Geometry check sheet. Reference: the model listing, model coordinates, mm. A direction names the side the tool comes from. Coordinates: 2 decimals unless noted, no trailing zeros. Loops run counter-clockwise (first coordinate to the right, second up) from the corner with the lowest first, then second, coordinate; pieces in that order, holes last. Notation, with made-up numbers: (-3.75, -16.5) - (49.25, -16.5) arc R20 cw to (49.25, 21.5) - close; hole circle Ø2 at (46.25, -2.75). An arc over 180 degrees is marked (long way). Write each question's results on one line, items separated by ' | '. Start each with the question number.
(1) Material ranges on probe 1 along Y at (x, z) = (0, -5); probe 2 along X at (y, z) = (-6, 16.5); probe 3 along Y at (x, z) = (-21, 3), recorded low to high.
(2) Mould release check, pull along X, two halves, no side actions. Record for faces 6 (the face through (0.21, -4.61, -5.48)), 7 (the face through (-22.5, -1, 13)), 8 (the face through (-21.486, -7.168, 11.315)): pulls with the +X half, pulls with the -X half, needs draft (parallel to the pull), parting line crosses it, or undercut.
(3) Sectioned sample at C-C (x = 27). Enter the section's corners in (y, z).
(4) Sectioned sample at A-A (z = 18). Enter the section's corners in (x, y).
(5) Go/stop test with flat-tipped pins: pin 1 Ø6 at (x, z) = (2.5, 15.5) entering from +Y; pin 2 Ø12 at (y, z) = (-6.5, 3) entering from -X (3 decimals); pin 3 Ø2 at (x, z) = (25, -1.5) entering from -Y; pin 4 Ø5 at (x, z) = (11.5, 26) entering from -Y. Record where each tip stops, or that it passes through.
(6) Sectioned sample at B-B (x = 7). Enter the section's corners in (y, z), plus the area to 3 significant figures.
(7) Sectioned sample at D-D (y = 18.5). Enter the section's corners in (x, z).
(8) Access from +Z, -Z, +X, -X, +Y, -Y to the whole of each face (thin tool, end or side, straight path). Record for faces 1 (the face through (-20.5, -1, 13)), 2 (the face through (22, -11.2, 13)), 3 (the face through (15.5, 12, 25)), 4 (the face through (-21.514, 7.1, 18.954)), 5 (the face through (0, 12.8, 13)).
from build123d import *

# Parameters (mm, degrees)
SM_BASE_FLANGE_1_DEPTH = 30
SKETCH_6_R             = 1
CUT_EXTRUDE_1_DEPTH    = 56.577333509
SKETCH_7_W             = 7
SKETCH_7_H             = 10
CUT_EXTRUDE_2_DEPTH    = 45.522466239
EXTRUDE_START          = 4
EXTRUDE_1_DEPTH        = 4
SKETCH_9_W             = 60
SKETCH_9_H             = 42
SKETCH_9_R             = 1.6
EXTRUDE_2_DEPTH        = 3
SKETCH_13_R            = 1
SKETCH_13_R_2          = 0.99
CUT_EXTRUDE_6_DEPTH    = 65.277401573
EXTRUDE_4_DEPTH        = 10


# Read off the part's stored shape, not the designer's step: 基体-法兰1
with BuildPart() as part:
    # 基体-法兰1 outline → 基体-法兰1 (new body)
    with BuildSketch(Plane.XY):
        with BuildLine():
            Line((-22.5, 9.8), (-22.5, -11.2))
            Line((-22.5, -11.2), (-20.5, -11.2))
            Line((-20.5, -11.2), (-20.5, 9.8))
            ThreePointArc((-20.5, 9.8), (-20.207106781, 10.507106781), (-19.5, 10.8))
            Line((-19.5, 10.8), (19.5, 10.8))
            ThreePointArc((19.5, 10.8), (20.207106781, 10.507106781), (20.5, 9.8))
            Line((20.5, 9.8), (20.5, -11.2))
            Line((20.5, -11.2), (22.5, -11.2))
            Line((22.5, -11.2), (22.5, 9.8))
            ThreePointArc((22.5, 9.8), (21.621320344, 11.921320344), (19.5, 12.8))
            Line((19.5, 12.8), (-19.5, 12.8))
            ThreePointArc((-19.5, 12.8), (-21.621320344, 11.921320344), (-22.5, 9.8))
        make_face()
    extrude(amount=SM_BASE_FLANGE_1_DEPTH)

    # 草图6 → 切除-拉伸1 (cut, through all)
    with BuildSketch(Plane.ZY.offset(22.5)):
        with BuildLine():
            Line((30, -7.692697161), (30, 6.292697161))
            ThreePointArc((30, 6.292697161), (23.007302839, -0.7), (30, -7.692697161))
        make_face()
        with Locations((3, 6.8)):
            Circle(SKETCH_6_R)
        with Locations((18, 6.8)):
            Circle(SKETCH_6_R)
        with Locations((18, -8.2)):
            Circle(SKETCH_6_R)
        with Locations((3, -8.2)):
            Circle(SKETCH_6_R)
    extrude(amount=-CUT_EXTRUDE_1_DEPTH, mode=Mode.SUBTRACT)

    # 草图7 → 切除-拉伸2 (cut, through all)
    with BuildSketch(Plane(origin=(0, 12.8, 0), x_dir=(1, 0, 0), z_dir=(0, 1, 0))):
        with Locations((12, -25)):
            Rectangle(SKETCH_7_W, SKETCH_7_H)
    extrude(amount=-CUT_EXTRUDE_2_DEPTH, mode=Mode.SUBTRACT)

    # 草图8 → 凸台-拉伸1 (add)
    with BuildSketch(Plane(origin=(0, 0, 0), x_dir=(-1, 0, 0), z_dir=(0, 0, -1)).offset(EXTRUDE_START)):
        with BuildLine():
            Line((-20.5, -11.2), (-20.5, 9.8))
            ThreePointArc((-20.5, 9.8), (-20.207106781, 10.507106781), (-19.5, 10.8))
            Line((-19.5, 10.8), (19.5, 10.8))
            ThreePointArc((19.5, 10.8), (20.207106781, 10.507106781), (20.5, 9.8))
            Line((20.5, 9.8), (20.5, -11.2))
            Line((20.5, -11.2), (22.5, -11.2))
            Line((22.5, -11.2), (22.5, 9.8))
            ThreePointArc((22.5, 9.8), (21.621320344, 11.921320344), (19.5, 12.8))
            Line((19.5, 12.8), (-19.5, 12.8))
            ThreePointArc((-19.5, 12.8), (-21.621320344, 11.921320344), (-22.5, 9.8))
            Line((-22.5, 9.8), (-22.5, -11.2))
            Line((-22.5, -11.2), (-20.5, -11.2))
        make_face()
    extrude(amount=-EXTRUDE_1_DEPTH)

    # 草图9 → 凸台-拉伸2 (add)
    with BuildSketch(Plane(origin=(0, 0, -4), x_dir=(-1, 0, 0), z_dir=(0, 0, -1))):
        with Locations((0, 0.802163953)):
            Rectangle(SKETCH_9_W, SKETCH_9_H)
        with Locations((-27, 17.802163953)):
            Circle(SKETCH_9_R, mode=Mode.SUBTRACT)
        with Locations((27, 17.802163953)):
            Circle(SKETCH_9_R, mode=Mode.SUBTRACT)
        with Locations((27, -16.197836047)):
            Circle(SKETCH_9_R, mode=Mode.SUBTRACT)
        with Locations((-27, -16.197836047)):
            Circle(SKETCH_9_R, mode=Mode.SUBTRACT)
        with Locations((0, 7.802163953)):
            Circle(SKETCH_9_R, mode=Mode.SUBTRACT)
        with Locations((7, 0.802163953)):
            Circle(SKETCH_9_R, mode=Mode.SUBTRACT)
        with Locations((0, -6.197836047)):
            Circle(SKETCH_9_R, mode=Mode.SUBTRACT)
        with Locations((-7, 0.802163953)):
            Circle(SKETCH_9_R, mode=Mode.SUBTRACT)
        with Locations((0, 0.802163953)):
            Circle(SKETCH_9_R, mode=Mode.SUBTRACT)
    extrude(amount=EXTRUDE_2_DEPTH)

    # 草图13 → 切除-拉伸6 (cut, through all)
    with BuildSketch(Plane(origin=(22.5, 0, 0), x_dir=(0, 0, -1), z_dir=(1, 0, 0))):
        with Locations(Location((-23.7, 7.3, 0), (0, 0, 90))):
            Circle(SKETCH_13_R)
        with Locations(Location((-10.48, 6.3, 0), (0, 0, 90))):
            Circle(SKETCH_13_R)
        with Locations(Location((-3.48, -0.7, 0), (0, 0, 90))):
            Circle(SKETCH_13_R)
        with Locations(Location((-23.7, -8.7, 0), (0, 0, 90))):
            Circle(SKETCH_13_R)
        with Locations(Location((-10.48, -7.7, 0), (0, 0, 90))):
            Circle(SKETCH_13_R_2)
    extrude(amount=-CUT_EXTRUDE_6_DEPTH, mode=Mode.SUBTRACT)

    # 草图17 → 凸台-拉伸4 (add, symmetric)
    with BuildSketch(Plane(origin=(0, 0, 0), x_dir=(1, 0, 0), z_dir=(0, 1, 0))):
        Polygon((-30, 4), (-22.5, 0), (-22.5, 4), align=None)
        Polygon((22.5, 0), (22.5, 4), (30, 4), align=None)
    extrude(amount=EXTRUDE_4_DEPTH, both=True)


solid = part.part
Outcome:
1) probe 1: y = -20.2 to -7.8, -4.6 to -0.8, 2.4 to 6.2, 9.4 to 21.8 | probe 2: x = -22.5 to -20.5, 20.5 to 22.5 | probe 3: y = -11.2 to -9.2, -7.2 to -1.58, 0.18 to 5.8, 7.8 to 12.4
2) face 6: undercut | face 7: pulls with the -X half | face 8: needs draft
3) outline: (-20.2, -7) - (-17.8, -7) - (-17.8, -4) - (-20.2, -4) - close; (-14.6, -7) - (16.2, -7) - (16.2, -4) - (10, -4) - (10, -2.4) - (-10, -2.4) - (-10, -4) - (-14.6, -4) - close; (19.4, -7) - (21.8, -7) - (21.8, -4) - (19.4, -4) - close
4) outline: (-22.5, -11.2) - (-20.5, -11.2) - (-20.5, -9.2) - (-22.5, -9.2) - close; (-22.5, -7.2) - (-20.5, -7.2) - (-20.5, 5.8) - (-22.5, 5.8) - close; (-22.5, 7.8) - (-20.5, 7.8) - (-20.5, 9.8) arc R1 cw to (-19.5, 10.8) - (19.5, 10.8) arc R1 cw to (20.5, 9.8) - (20.5, 7.8) - (22.5, 7.8) - (22.5, 9.8) arc R3 ccw to (19.5, 12.8) - (-19.5, 12.8) arc R3 ccw to (-22.5, 9.8) - close; (20.5, -11.2) - (22.5, -11.2) - (22.5, -9.2) - (20.5, -9.2) - close; (20.5, -7.2) - (22.5, -7.2) - (22.5, 5.8) - (20.5, 5.8) - close
5) pin 1: stops at y = 12.8 | pin 2: stops at x = -28.125 | pin 3: stops at y = -10 | pin 4: passes through
6) outline: (-20.2, -7) - (-0.8, -7) - (-0.8, -4) - (-20.2, -4) - close; (2.4, -7) - (21.8, -7) - (21.8, -4) - (12.8, -4) - (12.8, 30) - (10.8, 30) - (10.8, -4) - (2.4, -4) - close | area: 184 mm2
7) outline: (-30, -7) - (-28.44, -7) - (-28.44, -4) - (-30, -4) - close; (-25.56, -7) - (25.56, -7) - (25.56, -4) - (-25.56, -4) - close; (28.44, -7) - (30, -7) - (30, -4) - (28.44, -4) - close
8) face 1: +Z, -Y | face 2: +Z, +X, -X, -Y | face 3: +Z, +Y, -Y | face 4: +X, -X | face 5: +Z, +X, -X, +Y
